Geometry: final body of the model. Coordinates: model frame, mm. Give positions to 0.01 mm unless a question says otherwise; leave off trailing zeros. Loops run counter-clockwise (first coordinate to the right, second up) from the corner with the lowest first, then second, coordinate; pieces in that order, holes last. Notation, with made-up numbers: (-39.5, 21) - (-30.5, 21) arc R15 cw to (-30.5, 50) - close; hole circle Ø5 at (33, 64.5). An arc over 180 degrees is marked (long way). Use CSV: the item, a comma, the result in double quotes. Start each with the question number.
Autodesk Fusion 360 part; units mm, degrees
sketch "Sketch1" plane through (0, 0, 0) normal (0, 1, 0) x (1, 0, 0)
  line L0 (-127, -63.5) -> (127, -63.5)
  line L1 (127, -63.5) -> (127, 63.5)
  line L2 (127, 63.5) -> (-127, 63.5)
  line L3 (-127, 63.5) -> (-127, -63.5)
  circle A0 centre (-101.6, -38.1) radius 3.175
  circle A1 centre (-114.3, 50.8) radius 3.175
  circle A2 centre (-63.5, 25.4) radius 3.175
  circle A3 centre (-25.4, -12.7) radius 3.175
  circle A4 centre (25.4, -38.1) radius 3.175
  circle A5 centre (38.1, 12.7) radius 3.175
  circle A6 centre (12.7, 50.8) radius 3.175
  circle A7 centre (76.2, 38.1) radius 3.175
  circle A8 centre (88.9, -38.1) radius 6.35
  circle A9 centre (101.6, 12.7) radius 6.35
  circle A10 centre (-25.4, 38.1) radius 6.35
  circle A11 centre (-38.1, 12.7) radius 6.35
  circle A12 centre (-76.2, -38.1) radius 6.35
  circle A13 centre (-101.6, 25.4) radius 6.35
  circle A14 centre (-25.4, -50.8) radius 6.35
  circle A15 centre (38.1, 50.8) radius 6.35
  circle A16 centre (50.8, -25.4) radius 4.7625
  circle A17 centre (-63.5, -12.7) radius 4.7625
  circle A18 centre (-101.6, 0) radius 4.7625
  circle A19 centre (-76.2, 50.8) radius 4.7625
  circle A20 centre (101.6, 50.8) radius 4.7625
  circle A21 centre (114.3, -25.4) radius 4.7625
  circle A22 centre (63.5, -50.8) radius 4.7625
  circle A23 centre (0, -25.4) radius 4.7625
  dimension "d1" = 6.35
  dimension "d2" = 6.35
  dimension "d3" = 6.35
  dimension "d4" = 6.35
  dimension "d5" = 12.7
  dimension "d6" = 12.7
  dimension "d7" = 9.525
  dimension "d8" = 9.525
extrude "Extrude1" add sketch "Sketch1" along normal blind 25.4
Item 1: Mould query, pull axis X, two halves, no side actions, for faces 1 (the cylindrical face through (-32.234, 12.522, -15.132)), 2 (the flat face through (127, 13, 1)), 3 (the flat face through (-2, 25.4, -1)), 4 (the cylindrical face through (58.742, 12.522, 51.009)). Classes: pulls with the +X half, pulls with the -X half, needs draft (parallel to the pull), parting line crosses it, or undercut.
Item 2: Section D-D (x = -25.4). Output: boundary loops of the cut face in (y, z) (3 decimals).
Item 3: Ray query, probe 1 along X at (y, z) = (12.5, 25.4); probe 2 along X at (y, z) = (18.25, 50.8); probe 3 along Z at (x, y) = (-25.4, 17.75) (3 decimals). Return the intervals inside material, ascending.
Item 4: Section B-B (x = 12.7). Output: boundary loops of the cut face in (y, z) (3 decimals), plus the area to 3 significant figures.
Item 5: Section A-A (z = 50.8). Output: boundary loops of the cut face in (x, y).
Item 6: Section C-C (z = -12.7). Output: boundary loops of the cut face in (x, y) (3 decimals), plus the area to 3 significant figures.
Outcome:
1,face 1,"undercut"
1,face 2,"pulls with the +X half"
1,face 3,"needs draft"
1,face 4,"undercut"
2,outline,"(0, -63.5) - (25.4, -63.5) - (25.4, -44.45) - (0, -44.45) - close; (0, -31.75) - (25.4, -31.75) - (25.4, 9.525) - (0, 9.525) - close; (0, 15.875) - (25.4, 15.875) - (25.4, 44.45) - (0, 44.45) - close; (0, 57.15) - (25.4, 57.15) - (25.4, 63.5) - (0, 63.5) - close"
3,probe 1,"x = -127 to -4.76, 4.76 to 46.04, 55.56 to 109.54, 119.06 to 127"
3,probe 2,"x = -127 to -31.75, -19.05 to 58.74, 68.26 to 127"
3,probe 3,"z = -63.5 to -44.45, -31.75 to 9.525, 15.875 to 44.45, 57.15 to 63.5"
4,outline,"(0, -63.5) - (25.4, -63.5) - (25.4, -53.975) - (0, -53.975) - close; (0, -47.625) - (25.4, -47.625) - (25.4, 63.5) - (0, 63.5) - close"
4,area,"3,060 mm2"
5,outline,"(-127, 0) - (-31.75, 0) - (-31.75, 25.4) - (-127, 25.4) - close; (-19.05, 0) - (58.74, 0) - (58.74, 25.4) - (-19.05, 25.4) - close; (68.26, 0) - (127, 0) - (127, 25.4) - (68.26, 25.4) - close"
6,outline,"(-127, 0) - (-44.45, 0) - (-44.45, 25.4) - (-127, 25.4) - close; (-31.75, 0) - (34.925, 0) - (34.925, 25.4) - (-31.75, 25.4) - close; (41.275, 0) - (95.25, 0) - (95.25, 25.4) - (41.275, 25.4) - close; (107.95, 0) - (127, 0) - (127, 25.4) - (107.95, 25.4) - close"
6,area,"5,650 mm2"
